from build123d import *

# Parameters (mm, degrees)
SKETCH_1_R      = 1.5
SKETCH_1_W      = 4
SKETCH_1_H      = 8
SKETCH_1_R_2    = 4.1
SKETCH_1_R_3    = 11.1
EXTRUDE_6_DEPTH = 5


with BuildPart() as part:
    # 草图1 → 凸台-拉伸6 (new body)
    with BuildSketch(Plane(origin=(0, 0, 0), x_dir=(1, 0, 0), z_dir=(0, 1, 0))):
        Polygon((75, 150), (37.5, 150), (0, 150), (0, 0), (75, 0), align=None)
        with Locations((6, 10.5)):
            Circle(SKETCH_1_R, mode=Mode.SUBTRACT)
        with Locations((12.5, 10.5)):
            Rectangle(SKETCH_1_W, SKETCH_1_H, mode=Mode.SUBTRACT)
        with Locations((18.5, 10.5)):
            Circle(SKETCH_1_R, mode=Mode.SUBTRACT)
        with Locations((30.5, 10.5)):
            Circle(SKETCH_1_R, mode=Mode.SUBTRACT)
        with Locations((44.5, 10.5)):
            Circle(SKETCH_1_R, mode=Mode.SUBTRACT)
        with Locations((56.5, 10.5)):
            Circle(SKETCH_1_R, mode=Mode.SUBTRACT)
        with Locations((62.5, 10.5)):
            Rectangle(SKETCH_1_W, SKETCH_1_H, mode=Mode.SUBTRACT)
        with Locations((69, 10.5)):
            Circle(SKETCH_1_R, mode=Mode.SUBTRACT)
        with Locations((37.5, 132.25)):
            Circle(SKETCH_1_R_2, mode=Mode.SUBTRACT)
        with Locations((37.5, 113)):
            Circle(SKETCH_1_R_3, mode=Mode.SUBTRACT)
    extrude(amount=EXTRUDE_6_DEPTH)


solid = part.part
The model under review builds one solid part; all positions refer to its coordinate system, in mm. A direction names the side the tool comes from. Coordinates: 2 decimals unless noted, no trailing zeros. Loops run counter-clockwise (first coordinate to the right, second up) from the corner with the lowest first, then second, coordinate; pieces in that order, holes last.
(1) Consider section B-B, the plane x = 6. Give the boundary of the cut face in (y, z), plus the area to 3 significant figures.
Determined:
outline: (0, -150) - (5, -150) - (5, -12) - (0, -12) - close; (0, -9) - (5, -9) - (5, 0) - (0, 0) - close
area: 735 mm2
(2) Consider section C-C, the plane y = 2.25. Give the number of separate pieces and of enclosed holes in the cut face, plus the area to 3 significant figures.
Determined:
separate pieces: 1
enclosed holes: 10
area: 10,700 mm2
(3) Consider section A-A, the plane z = -132.25. Give the boundary of the cut face in (x, y), plus the area to 3 significant figures.
Determined:
outline: (0, 0) - (33.4, 0) - (33.4, 5) - (0, 5) - close; (41.6, 0) - (75, 0) - (75, 5) - (41.6, 5) - close
area: 334 mm2
(4) Consider section D-D, the plane x = 44.5. Give the boundary of the cut face in (y, z), plus the area to 3 significant figures.
Determined:
outline: (0, -150) - (5, -150) - (5, -121.61) - (0, -121.61) - close; (0, -104.39) - (5, -104.39) - (5, -12) - (0, -12) - close; (0, -9) - (5, -9) - (5, 0) - (0, 0) - close
area: 649 mm2
(5) Tool access review of faces 1 (the flat face through (75, 2, -74)), 2 (the flat face through (12, 2, -14.5)): name each direction out of +Z, -Z, +X, -X, +Y, -Y from which nothing blocks a thin tool from reaching the whole face with its end or side.
Determined:
face 1: +Z, -Z, +X, +Y, -Y
face 2: +Y, -Y
(6) Wall thickness on L1, parallel to Z at x = 37.5, y = 2.1; L2, parallel to Z at x = 44.5, y = 2.6; L3, parallel to Z at x = 57.5, y = 0.3: over which ranges is each line inside the solid? List them lowest first.
Determined:
L1: z = -150 to -136.35, -128.15 to -124.1, -101.9 to 0
L2: z = -150 to -121.61, -104.39 to -12, -9 to 0
L3: z = -150 to -11.62, -9.38 to 0
(7) Draft analysis for pull direction Z (two halves, no side actions). For faces 3 (the flat face through (0, 2, -76)), 4 (the flat face through (38, 2, -150)), 5 (the cylindrical face through (35.094, 2.465, -102.164)), state which applies: +Z half, -Z half, draft (parallel to the pull), parting line (faces both ways), or undercut.
Determined:
face 3: draft
face 4: -Z half
face 5: undercut
